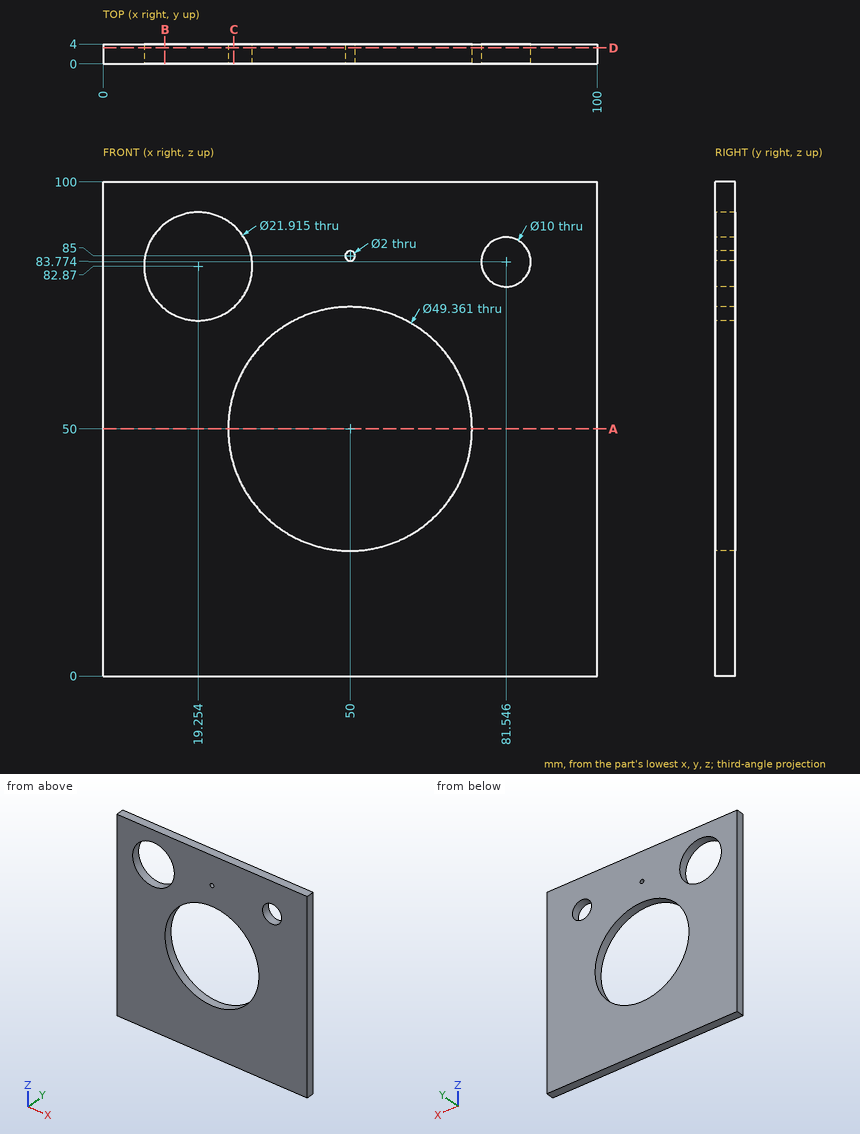
Here's the drawing with two shaded views (mm, measured from the low corner). I have some questions. Give positions to 0.01 mm unless a question says otherwise; leave off trailing zeros. Loops run counter-clockwise (first coordinate to the right, second up) from the corner with the lowest first, then second, coordinate; pieces in that order, holes last. Notation, with made-up numbers: (31.25, -32) - (81.25, -32) arc R27 ccw to (81.25, 2) - close; hole circle Ø9 at (-18, 72.5). An arc over 180 degrees is marked (long way). Return JSON: item names as keys, results as strings.
1. I'm going to push a flat-ended pin straight in: pin 1 Ø13 at (x, z) = (19.25, 82.87) entering from -Y. Where does the tip first touch, or does it pass through?
Output values:
{"pin 1": "passes through"}
2. I want a section at A-A on z = 50. Please give me the cut outline in (x, y).
Output values:
{"outline": "(0, 0) - (25.32, 0) - (25.32, 4) - (0, 4) - close; (74.68, 0) - (100, 0) - (100, 4) - (74.68, 4) - close"}
3. I want a section at B-B on x = 12.5. Please give me the cut outline in (y, z).
Output values:
{"outline": "(0, 0) - (4, 0) - (4, 74.24) - (0, 74.24) - close; (0, 91.5) - (4, 91.5) - (4, 100) - (0, 100) - close"}
4. I want a section at C-C on x = 26.5. Please give me the cut outline in (y, z), and give its area (3 significant figures).
Output values:
{"outline": "(0, 0) - (4, 0) - (4, 42.46) - (0, 42.46) - close; (0, 57.54) - (4, 57.54) - (4, 74.65) - (0, 74.65) - close; (0, 91.09) - (4, 91.09) - (4, 100) - (0, 100) - close", "area": "274 mm²"}
5. If I drill on line 1 (Z direction, x = 50, y = 0.95); line 2 (X direction, y = 2.35, z = 85) (1 decimal); line 3 (Z direction, x = 42.5, y = 0.3), over which ranges is the centre line in solid material (lowest first)?
Output values:
{"line 1": "z = 0 to 25.32, 74.68 to 84, 86 to 100", "line 2": "x = 0 to 8.5, 30 to 49, 51 to 76.7, 86.4 to 100", "line 3": "z = 0 to 26.49, 73.51 to 100"}
6. I want a section at D-D on y = 3.2. Please give me the cut outline in (x, z) (1 decimal).
Output values:
{"outline": "(0, 0) - (100, 0) - (100, 100) - (0, 100) - close; hole circle Ø21.9 at (19.3, 82.9); hole circle Ø49.4 at (50, 50); hole circle Ø2 at (50, 85); hole circle Ø10 at (81.5, 83.8)"}
